Verification items for the finished model (mm, model axes). Face numbers are marked on the shaded views. A direction names the side the tool comes from. Round coordinates to 2 decimals unless told otherwise and drop trailing zeros. Order: outer loops, then holes, each group sorted by start corner. A loop starts at its lowest first (then second) coordinate and runs counter-clockwise, first axis right, second up.
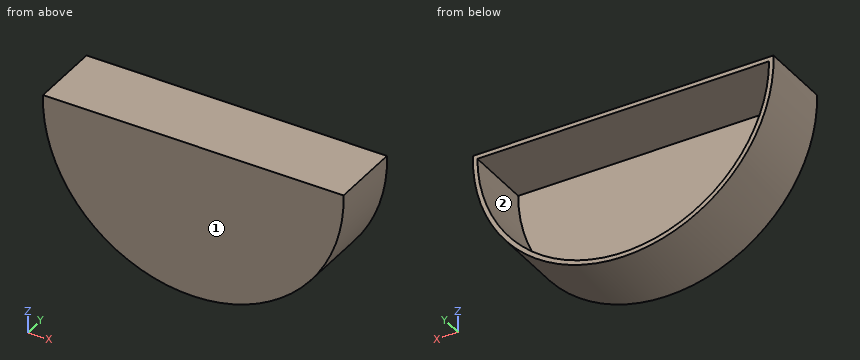
```python
from build123d import *

# Parameters (mm, degrees)
BOSS_EXTRUDE2_DEPTH = 6
BOSS_EXTRUDE3_DEPTH = 0.4


with BuildPart() as part:
    # Sketch3 → Boss-Extrude2 (new body)
    with BuildSketch(Plane(origin=(0, 0, 0), x_dir=(1, 0, 0), z_dir=(0, 1, 0))):
        with BuildLine():
            Line((-13.39402852, -0.4), (13.39402852, -0.4))
            ThreePointArc((13.39402852, -0.4), (0, 13.4), (-13.39402852, -0.4))
        make_face()
        with BuildLine():
            Line((-13, 0), (13, 0))
            ThreePointArc((13, 0), (0, 13), (-13, 0))
        make_face(mode=Mode.SUBTRACT)
    extrude(amount=BOSS_EXTRUDE2_DEPTH)

    # Sketch4 → Boss-Extrude3 (add)
    with BuildSketch(Plane.XZ):
        with BuildLine():
            Line((-13.39402852, 0.4), (13.39402852, 0.4))
            ThreePointArc((13.39402852, 0.4), (0, -13.4), (-13.39402852, 0.4))
        make_face()
    extrude(amount=BOSS_EXTRUDE3_DEPTH)


solid = part.part
```
1) Sectioned sample at A-A on x = 0. Record the cut outline in (y, z), then the cut area to 3 significant figures.
2) Scan lines: probe 1 along Y at (x, z) = (-6, -2.75); probe 2 along Z at (x, y) = (10.75, 4.75); probe 3 along Z at (x, y) = (6, 0.25). Record each from-to range of solid material in increasing order.
3) Go/stop test with flat-tipped pins: pin 1 Ø3 at (x, y) = (2.5, 3.5) entering from -Z; pin 2 Ø1 at (x, z) = (2.5, -12) entering from +Y; pin 3 Ø1 at (y, z) = (5, -7.5) entering from -X. Record where each tip stops, or that it passes through.
4) Sectioned sample at B-B on z = -2.75. Record the cut outline in (x, y).
5) Tool access check on the marked faces 1 and 2. Record the directions out of +Z, -Z, +X, -X, +Y, -Y that give a thin tool (end or side, any length) a straight path to the whole face; none if there is none.
Returned:
1. outline: (-0.4, -13.4) - (6, -13.4) - (6, -13) - (0, -13) - (0, 0) - (6, 0) - (6, 0.4) - (-0.4, 0.4) - close
1. area: 10.3 mm2
2. probe 1: y = -0.4 to 0
2. probe 2: z = -8 to -7.31, 0 to 0.4
2. probe 3: z = -11.98 to -11.53, 0 to 0.4
3. pin 1: stops at z = -13.36
3. pin 2: stops at y = 0
3. pin 3: stops at x = -11.43
4. outline: (-13.11, -0.4) - (13.11, -0.4) - (13.11, 6) - (12.71, 6) - (12.71, 0) - (-12.71, 0) - (-12.71, 6) - (-13.11, 6) - close
5. face 1: +Z, -Z, +X, -X, -Y
5. face 2: +Y
